Could you check a few things on this model? Use its own coordinates, in mm. A direction names the side the tool comes from. Give positions to 0.01 mm unless a question says otherwise; leave off trailing zeros. Order: outer loops, then holes, each group sorted by start corner. A loop starts at its lowest first (then second) coordinate and runs counter-clockwise, first axis right, second up. Notation, with made-up numbers: (46, 25.25) -> (90, 25.25) arc R19 ccw to (90, 41.25) -> close; hole circle Ø9 at (2, 35). An arc over 180 degrees is marked (long way). One line per item, written item: value.
Autodesk Inventor part; units mm, degrees
ref_plane "YZ Plane" through (0, 0, 0) normal (1, 0, 0) x (0, 1, 0)
ref_plane "XZ Plane" through (0, 0, 0) normal (0, 1, 0) x (-1, 0, 0)
ref_plane "XY Plane" through (0, 0, 0) normal (0, 0, 1) x (1, 0, 0)
sketch "Skizze1" plane through (0, 0, 0) normal (0, 0, 1) x (1, 0, 0)
  line L0 (0, 0) -> (32, 0)
  line L1 (32, 0) -> (32, 59)
  line L2 (32, 59) -> (0, 59)
  line L3 (0, 59) -> (0, 0)
  dimension "d0" = 32
  dimension "d1" = 59
extrude "Extrusion1" add sketch "Skizze1" against normal blind 31
sketch "Skizze2" plane through (0, 0, -31) normal (0, 0, -1) x (-1, 0, 0)
  line L0 (-2, 57) -> (-30, 57)
  line L1 (-30, 57) -> (-30, 2)
  line L2 (-30, 2) -> (-2, 2)
  line L3 (-2, 2) -> (-2, 57)
  line L4 (0, 59) -> (-32, 59) construction
  line L5 (-32, 59) -> (-32, 0) construction
  point P0 (0, 0)
  dimension "d4" = 2
  dimension "d5" = 2
  dimension "d6" = 2
  dimension "d7" = 2
extrude "Extrusion2" cut sketch "Skizze2" against normal blind 28.5
sketch "Skizze8" plane through (0, 0, -2.5) normal (0, 0, -1) x (-1, 0, 0)
  line L0 (-6, 12) -> (-26, 12)
  line L1 (-26, 12) -> (-26, 15)
  line L2 (-26, 15) -> (-6, 15)
  line L3 (-6, 15) -> (-6, 12)
  line L4 (-2, 2) -> (-30, 2) construction
  circle A0 centre (-4.61, 4.57) radius 3 construction
  line L5 (-6, 43.5) -> (-26, 43.5)
  line L6 (-26, 43.5) -> (-26, 40.5)
  line L7 (-26, 40.5) -> (-6, 40.5)
  line L8 (-6, 40.5) -> (-6, 43.5)
  circle A1 centre (-4.61, 50.29) radius 3 construction
  line L9 (-30, 57) -> (-2, 57)
  point P0 (0, 0)
  point P1 (-16, 12)
  point P2 (-16, 2)
  point P3 (-16, 2)
  point P4 (-16, 40.5)
  dimension "d43" = 3
  dimension "d44" = 20
  dimension "d46" = 3
  dimension "d47" = 20
  dimension "d71" = 10
  dimension "d72" = 13.5
extrude "Extrusion5" cut sketch "Skizze8" against normal through all
sketch "Skizze9" plane through (0, 0, 0) normal (0, -1, 0) x (1, 0, 0)
  line L0 (2, -5.5) -> (3.0624, -5.5) construction
  line L1 (17.5, -12.3) -> (9.5, -12.3)
  line L2 (9.5, -12.3) -> (9.5, -9.3)
  line L3 (9.5, -9.3) -> (17.5, -9.3)
  line L4 (17.5, -9.3) -> (17.5, -12.3)
  line L5 (0, 0) -> (32, 0) construction
  line L6 (2, -2.5) -> (30, -2.5)
  line L7 (2, -31) -> (2, -2.5)
  point P0 (13.5, -9.3)
  point P1 (16, 0)
  point P2 (6.1576, -2)
  point P3 (20.8424, -2)
  point P4 (30, -2.5)
  dimension "d54" = 8
  dimension "d55" = 3
  dimension "d70" = 6.8
  dimension "d81" = 7.5
extrude "Extrusion6" cut sketch "Skizze9" against normal up to surface (2 mm away)
fillet "Rundung1" radius 2 4 edges at (32, 0, -15.5) (0, 0, -15.5) (0, 59, -15.5) (32, 59, -15.5)
fillet "Rundung2" radius 2 2 edges at (16, 15, -2.5) (16, 40.5, -2.5)
fillet "Rundung3" radius 2 2 edges at (16, 12, 0) (16, 43.5, 0)
sketch "Skizze11" plane through (0, 0, -2.5) normal (0, 0, -1) x (-1, 0, 0)
  point P0 (0, 0)
  point P1 (-22.39, 5)
  point P2 (-22.39, 5)
  point P3 (-4.61, 5)
  point P4 (-4.61, 5)
  point P5 (-22.39, 50.72)
  point P6 (-22.39, 50.72)
  point P7 (-4.61, 50.72)
  dimension "d82" = 4.61
  dimension "d83" = 5
  dimension "d84" = 45.72
  dimension "d85" = 17.78
hole "Bohrung4" at (22.39, 5, -2.5) at (4.61, 5, -2.5) at (22.39, 50.72, -2.5) at (4.61, 50.72, -2.5) direction (0, 0, 1) diameter 2.6 end through all
properties part number "bottom"
1) For faces 1 (the flat face through (26, 42, -1)), 2 (the flat face through (16, 2, -17)), 3 (the cylindrical face through (15.86, 44.07, -0.6)), 4 (the flat face through (14, 1, -12.3)), which set-ups out of +Z, -Z, +X, -X, +Y, -Y let a thin tool reach every point of the face, with its end or its side?
Answer below:
face 1: none
face 2: -Z
face 3: +Z
face 4: -Y
2) Suppose I cut it at A-A, the plane y = 4.5. Write out the boundary of the cut face in (x, z), then the cut area to 3 significant figures.
Answer below:
outline: (0, -31) -> (2, -31) -> (2, -2.5) -> (3.41, -2.5) -> (3.41, 0) -> (0, 0) -> close; (5.81, -2.5) -> (21.19, -2.5) -> (21.19, 0) -> (5.81, 0) -> close; (23.59, -2.5) -> (30, -2.5) -> (30, -31) -> (32, -31) -> (32, 0) -> (23.59, 0) -> close
area: 182 mm2
3) Suppose I cut it at C-C, the plane z = -26.5. Write out the boundary of the cut face in (x, y).
Answer below:
outline: (0, 2) arc R2 ccw to (2, 0) -> (30, 0) arc R2 ccw to (32, 2) -> (32, 57) arc R2 ccw to (30, 59) -> (2, 59) arc R2 ccw to (0, 57) -> close; hole (2, 2) -> (30, 2) -> (30, 57) -> (2, 57) -> close
4) Suppose I cut it at D-D, the plane x = 22.39. Write out the boundary of the cut face in (y, z).
Answer below:
outline: (0, -31) -> (2, -31) -> (2, -2.5) -> (3.7, -2.5) -> (3.7, 0) -> (0, 0) -> close; (6.3, -2.5) -> (12, -2.5) -> (12, -2) arc R2 ccw to (10, 0) -> (6.3, 0) -> close; (15, -0.5) arc R2 ccw to (17, -2.5) -> (38.5, -2.5) arc R2 ccw to (40.5, -0.5) -> (40.5, 0) -> (15, 0) -> close; (43.5, -2.5) -> (49.42, -2.5) -> (49.42, 0) -> (45.5, 0) arc R2 ccw to (43.5, -2) -> close; (52.02, -2.5) -> (57, -2.5) -> (57, -31) -> (59, -31) -> (59, 0) -> (52.02, 0) -> close
5) For P1, Ø2, axis at y = 1, z = -10.5, coming from the +X side; P2, Ø14, axis at x = 17.5, y = 27.5, coming from the -Z side, each with a flat end and sliding along its axis, tell me the tip position at first contact or that it passes through.
Answer below:
P1: stops at x = 32
P2: stops at z = -2.5
6) Suppose I cut it at B-B, the plane x = 4.61. Write out the boundary of the cut face in (y, z).
Answer below:
outline: (0, -31) -> (2, -31) -> (2, -2.5) -> (3.7, -2.5) -> (3.7, 0) -> (0, 0) -> close; (6.3, -2.5) -> (49.42, -2.5) -> (49.42, 0) -> (6.3, 0) -> close; (52.02, -2.5) -> (57, -2.5) -> (57, -31) -> (59, -31) -> (59, 0) -> (52.02, 0) -> close
7) If I drill on line 1 along X through (y, z) = (50.72, -0.55); line 2 along Y through (x, z) = (4.61, -1.5); line 3 along Y through (x, z) = (19.5, -9), over which ranges is the centre line in solid material (lowest first)?
Answer below:
line 1: x = 0 to 3.31, 5.91 to 21.09, 23.69 to 32
line 2: y = 0 to 3.7, 6.3 to 49.42, 52.02 to 59
line 3: y = 0 to 2, 57 to 59
8) We'd pull the mould along Z, two halves only. Please class faces 5 (the flat face through (9.5, 1, -11)), 6 (the cylindrical face through (15.86, 39.93, -1.9)), 7 (the cylindrical face through (21.1, 4.83, -1.23)): +Z half, -Z half, draft (parallel to the pull), parting line (faces both ways), or undercut.
Answer below:
face 5: undercut
face 6: -Z half
face 7: draft
